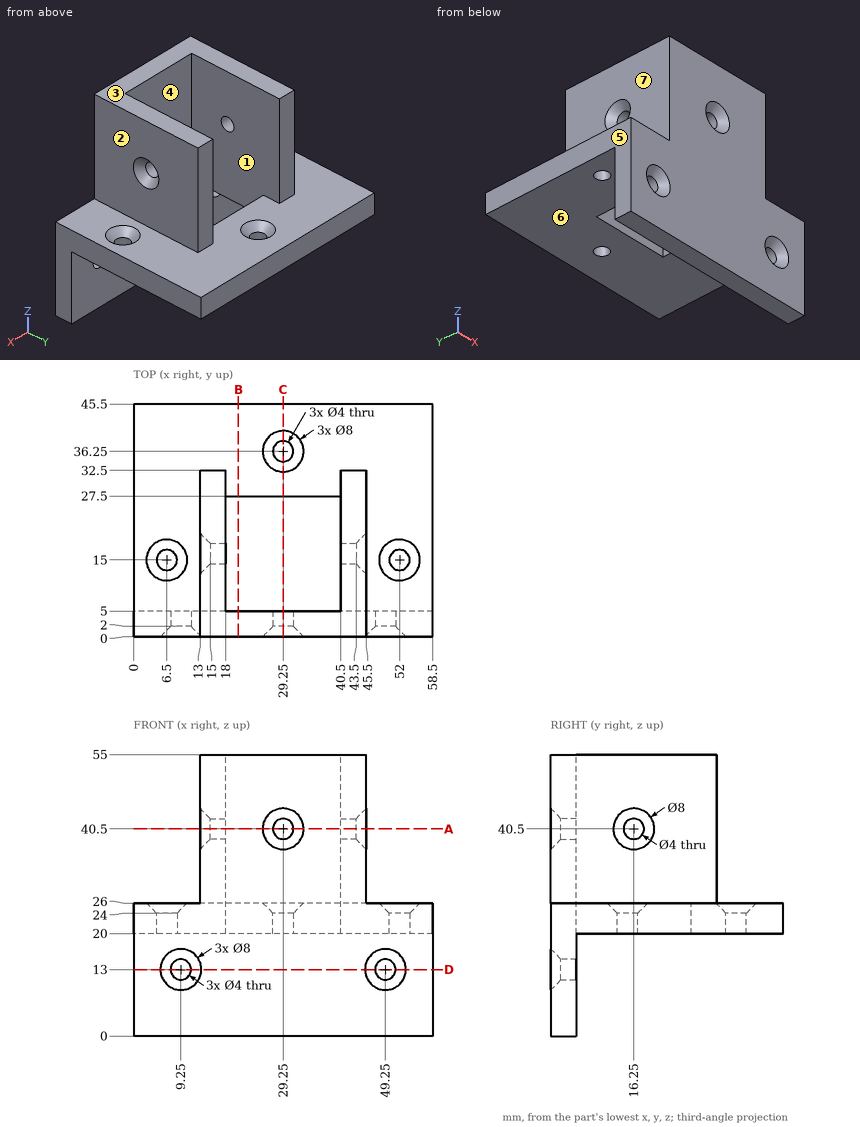
Geometry: see drawing. Coordinates: mm, zero at the bounding-box minimum. A direction names the side the tool comes from. Round coordinates to 2 decimals unless told otherwise and drop trailing zeros. Loops run counter-clockwise (first coordinate to the right, second up) from the corner with the lowest first, then second, coordinate; pieces in that order, holes last. Notation, with made-up numbers: (72.25, 89.25) -> (119.25, 89.25) arc R24 ccw to (119.25, 125.25) -> close; hole circle Ø10 at (53.5, 21.25). An arc over 180 degrees is marked (long way). One line per question, with ' | ' between items. Start each with the question number.
1. Section C-C on x = 29.25. Output: boundary loops of the cut face in (y, z).
2. Line query: line 1 along Y through (x, z) = (29, 22); line 2 along X through (y, z) = (4, 13); line 3 along Z through (x, y) = (16, 16). Output: solid intervals per line, ascending. Write a range as [from, to].
3. Section B-B on x = 20.5. Output: boundary loops of the cut face in (y, z), and give its area (3 significant figures).
4. Contact query for flat-ended pins moving along their axis: pin 1 (12 mm diameter, centred on x = 19, y = 35, fed in from -Z); pin 2 (10 mm diameter, centred on y = 33, z = 29.5, fed in from +X); pin 3 (2.5 mm diameter, centred on x = 52, y = 15, fed in from +Z); pin 4 (8 mm diameter, centred on x = 20, z = 47, fed in from +Y). Output: stop coordinate, or through.
5. Mould query, pull axis X, two halves, no side actions, for the marked faces 1, 2, 3 and 4. Classes: pulls with the +X half, pulls with the -X half, needs draft (parallel to the pull), parting line crosses it, or undercut.
6. Section D-D on z = 13. Output: boundary loops of the cut face in (x, y), and give its area (4 significant figures).
7. Section A-A on z = 40.5. Output: boundary loops of the cut face in (x, y).
8. Set-up query: the marked faces 5, 6 and 7. Return all of +Z, -Z, +X, -X, +Y, -Y with unobstructed straight access to the full face (end or side cutting, diameter ignored); none if empty.
Returned:
1) outline: (0, 0) -> (5, 0) -> (5, 38.5) -> (2, 38.5) -> (0, 36.5) -> close; (0, 44.5) -> (2, 42.5) -> (5, 42.5) -> (5, 55) -> (0, 55) -> close; (27.5, 20) -> (34.25, 20) -> (34.25, 24) -> (32.25, 26) -> (27.5, 26) -> close; (38.25, 20) -> (45.5, 20) -> (45.5, 26) -> (40.25, 26) -> (38.25, 24) -> close
2) line 1: y = [0, 5], [27.5, 34.27], [38.23, 45.5] | line 2: x = [0, 7.25], [11.25, 47.25], [51.25, 58.5] | line 3: z = [20, 38.52], [42.48, 55]
3) outline: (0, 0) -> (5, 0) -> (5, 55) -> (0, 55) -> close; (27.5, 20) -> (45.5, 20) -> (45.5, 26) -> (27.5, 26) -> close | area: 383 mm2
4) pin 1: stops at z = 20 | pin 2: stops at x = 58.5 | pin 3: passes through | pin 4: stops at y = 32.5
5) face 1: undercut | face 2: pulls with the +X half | face 3: needs draft | face 4: undercut
6) outline: (0, 0) -> (5.25, 0) -> (7.25, 2) -> (7.25, 5) -> (0, 5) -> close; (11.25, 2) -> (13.25, 0) -> (45.25, 0) -> (47.25, 2) -> (47.25, 5) -> (11.25, 5) -> close; (51.25, 2) -> (53.25, 0) -> (58.5, 0) -> (58.5, 5) -> (51.25, 5) -> close | area: 244.5 mm2
7) outline: (13, 0) -> (25.25, 0) -> (27.25, 2) -> (27.25, 5) -> (18, 5) -> (18, 14.25) -> (15, 14.25) -> (13, 12.25) -> close; (13, 20.25) -> (15, 18.25) -> (18, 18.25) -> (18, 32.5) -> (13, 32.5) -> close; (31.25, 2) -> (33.25, 0) -> (45.5, 0) -> (45.5, 12.25) -> (43.5, 14.25) -> (40.5, 14.25) -> (40.5, 5) -> (31.25, 5) -> close; (40.5, 18.25) -> (43.5, 18.25) -> (45.5, 20.25) -> (45.5, 32.5) -> (40.5, 32.5) -> close
8) face 5: +Z, -Z, -X, +Y, -Y | face 6: -Z, +X, -X, +Y | face 7: +Z, -X, +Y, -Y
